Here's how the part is built. I have some questions about the finished solid (model axes, mm). A direction names the side the tool comes from. Coordinates: 2 decimals unless noted, no trailing zeros. Loops run counter-clockwise (first coordinate to the right, second up) from the corner with the lowest first, then second, coordinate; pieces in that order, holes last. Notation, with made-up numbers: (13, 83) - (45, 83) arc R31 cw to (45, 118) - close; hole circle Ø2 at (-13.75, -16.5). An arc over 180 degrees is marked (long way). Use a Markdown table: item, result.
```python
from build123d import *

# Parameters (mm, degrees)
SKETCH_1_W               = 60
SKETCH_1_H               = 3
EXTRUDE_1_DEPTH          = 65
SKETCH_2_W               = 40
SKETCH_2_H               = 3.5
EXTRUDE_2_DEPTH          = 46
EXTRUDE_3_DEPTH          = 3.5
SKETCH_5_W               = 35
SKETCH_5_H               = 17
EXTRUDE_4_DEPTH          = 3
EXTRUDE_START            = 3
SKETCH_6_W               = 35
SKETCH_6_H               = 17
SKETCH_6_W_2             = 20
SKETCH_6_H_2             = 3.5
EXTRUDE_5_DEPTH          = 3
SKETCH_7_W               = 36
SKETCH_7_H               = 10
SKETCH_7_W_2             = 10
SKETCH_7_H_2             = 65
EXTRUDE_6_DEPTH          = 60
SKETCH_8_W               = 66
SKETCH_8_H               = 111
EXTRUDE_7_DEPTH          = 10
SKETCH_9_W               = 15
SKETCH_9_H               = 10
EXTRUDE_8_DEPTH          = 110
SKETCH_10_W              = 36
SKETCH_10_H              = 70
CUT_EXTRUDE_2_DEPTH      = 15
SKETCH_13_W              = 221
SKETCH_13_H              = 10
EXTRUDE_9_DEPTH          = 10
SKETCH_14_W              = 221
SKETCH_14_H              = 10
EXTRUDE_10_DEPTH         = 10
SKETCH_15_W              = 86
SKETCH_15_H              = 10
EXTRUDE_11_DEPTH         = 10
CHAMFER_1_SIZE           = 30
CHAMFER_2_SIZE           = 30
CUT_EXTRUDE_3_DEPTH      = 15
CUT_EXTRUDE_3_DEPTH_BACK = 75
SKETCH_16_R              = 2.1
CHAMFER_3_SIZE           = 5


with BuildPart() as part:
    # 草图1 → 凸台-拉伸1 (new body)
    with BuildSketch(Plane.XY):
        with Locations((0, -32)):
            Rectangle(SKETCH_1_W, SKETCH_1_H)
        with BuildLine():
            Line((-20, -24), (-20, -28))
            Line((-20, -28), (-20, -30))
            Line((-20, -30), (20, -30))
            Line((20, -30), (20, -28))
            Line((20, -28), (20, -24))
            ThreePointArc((20, -24), (21.171572875, -21.171572875), (24, -20))
            Line((24, -20), (28, -20))
            Line((28, -20), (30, -20))
            Line((30, -20), (30, -30.5))
            Line((30, -30.5), (-30, -30.5))
            Line((-30, -30.5), (-30, -20))
            Line((-30, -20), (-28, -20))
            Line((-28, -20), (-24, -20))
            ThreePointArc((-24, -20), (-21.171572875, -21.171572875), (-20, -24))
        make_face()
    extrude(amount=EXTRUDE_1_DEPTH)

    # 草图2 → 凸台-拉伸2 (add)
    with BuildSketch(Plane(origin=(0, 0, 0), x_dir=(-1, 0, 0), z_dir=(0, 0, -1))):
        with Locations((0, -31.75)):
            Rectangle(SKETCH_2_W, SKETCH_2_H)
    extrude(amount=EXTRUDE_2_DEPTH)

    # 草图4 → 凸台-拉伸3 (add)
    with BuildSketch(Plane.XZ.offset(33.5)):
        Polygon((20, -46), (30, -46), (30, -26), (20, -26), (-30, -26), (-30, -46), align=None)
    extrude(amount=-EXTRUDE_3_DEPTH)

    # 草图5 → 凸台-拉伸4 (add)
    with BuildSketch(Plane.ZY.offset(30)):
        with BuildLine():
            Line((-46, -26.5), (-46, -33.5))
            Line((-46, -33.5), (-26, -33.5))
            Line((-26, -33.5), (-26, 8.5))
            Line((-26, 8.5), (56.193548387, -33.5))
            Line((56.193548387, -33.5), (65, -20))
            Line((65, -20), (-26, 26.5))
            Line((-26, 26.5), (-96, 26.5))
            ThreePointArc((-96, 26.5), (-105, 17.5), (-96, 8.5))
            Line((-96, 8.5), (-96, -8.5))
            ThreePointArc((-96, -8.5), (-105, -17.5), (-96, -26.5))
            Line((-96, -26.5), (-46, -26.5))
        make_face()
        with Locations((-63.5, 0)):
            Rectangle(SKETCH_5_W, SKETCH_5_H, mode=Mode.SUBTRACT)
    extrude(amount=EXTRUDE_4_DEPTH)

    # 草图6 → 凸台-拉伸5 (add)
    # profile 1 of 3: a face of its own
    with BuildSketch(Plane(origin=(30, 0, 0), x_dir=(0, 0, -1), z_dir=(1, 0, 0)).offset(EXTRUDE_START)):
        Polygon((26, 8.5), (26, 26.5), (-65, -20), (-56.193548387, -33.5), align=None)
    # profile 2 of 3: a face of its own
    with BuildSketch(Plane(origin=(30, 0, 0), x_dir=(0, 0, -1), z_dir=(1, 0, 0)).offset(EXTRUDE_START)):
        with BuildLine():
            Line((96, 26.5), (46, 26.5))
            Line((46, 26.5), (26, 26.5))
            Line((26, 26.5), (26, 8.5))
            Line((26, 8.5), (26, -30))
            Line((26, -30), (46, -30))
            Line((46, -30), (46, -26.5))
            Line((46, -26.5), (96, -26.5))
            ThreePointArc((96, -26.5), (105, -17.5), (96, -8.5))
            Line((96, -8.5), (96, 8.5))
            ThreePointArc((96, 8.5), (105, 17.5), (96, 26.5))
        make_face()
        with Locations((63.5, 0)):
            Rectangle(SKETCH_6_W, SKETCH_6_H, mode=Mode.SUBTRACT)
    # profile 3 of 3: a face of its own
    with BuildSketch(Plane(origin=(30, 0, 0), x_dir=(0, 0, -1), z_dir=(1, 0, 0)).offset(EXTRUDE_START)):
        with Locations((36, -31.75)):
            Rectangle(SKETCH_6_W_2, SKETCH_6_H_2)
    extrude(amount=-EXTRUDE_5_DEPTH)

    # 草图7 → 凸台-拉伸6 (add)
    with BuildSketch(Plane.XZ.offset(33.5)):
        with Locations((0, -41)):
            Rectangle(SKETCH_7_W, SKETCH_7_H)
        with Locations((-25, 32.5)):
            Rectangle(SKETCH_7_W_2, SKETCH_7_H_2)
        with Locations((25, 32.5)):
            Rectangle(SKETCH_7_W_2, SKETCH_7_H_2)
    extrude(amount=EXTRUDE_6_DEPTH)

    # 草图8 → 凸台-拉伸7 (add)
    with BuildSketch(Plane.XZ.offset(93.5)):
        with Locations((0, 9.5)):
            Rectangle(SKETCH_8_W, SKETCH_8_H)
    extrude(amount=EXTRUDE_7_DEPTH)

    # 草图9 → 凸台-拉伸8 (add)
    with BuildSketch(Plane(origin=(0, 0, -46), x_dir=(-1, 0, 0), z_dir=(0, 0, -1))):
        with Locations((25.5, -98.5)):
            Rectangle(SKETCH_9_W, SKETCH_9_H)
        with Locations((-25.5, -98.5)):
            Rectangle(SKETCH_9_W, SKETCH_9_H)
    extrude(amount=EXTRUDE_8_DEPTH)

    # 草图10 → 切除-拉伸2 (cut)
    with BuildSketch(Plane(origin=(0, 0, -46), x_dir=(-1, 0, 0), z_dir=(0, 0, -1))):
        with Locations((0, -68.5)):
            Rectangle(SKETCH_10_W, SKETCH_10_H)
    extrude(amount=-CUT_EXTRUDE_2_DEPTH, mode=Mode.SUBTRACT)

    # 草图13 → 凸台-拉伸9 (add)
    with BuildSketch(Plane.ZY.offset(33)):
        with Locations((-45.5, -98.5)):
            Rectangle(SKETCH_13_W, SKETCH_13_H)
    extrude(amount=EXTRUDE_9_DEPTH)

    # 草图14 → 凸台-拉伸10 (add)
    with BuildSketch(Plane(origin=(33, 0, 0), x_dir=(0, 0, -1), z_dir=(1, 0, 0))):
        with Locations((45.5, -98.5)):
            Rectangle(SKETCH_14_W, SKETCH_14_H)
    extrude(amount=EXTRUDE_10_DEPTH)

    # 草图15 → 凸台-拉伸11 (add)
    with BuildSketch(Plane.XY.offset(65)):
        with Locations((0, -98.5)):
            Rectangle(SKETCH_15_W, SKETCH_15_H)
    extrude(amount=EXTRUDE_11_DEPTH)

    # 倒角1
    chamfer_1_edges = [part.edges().sort_by_distance(p)[0] for p in [
        (25, -93.5, 0),
    ]]
    chamfer(chamfer_1_edges, length=CHAMFER_1_SIZE)

    # 倒角2
    chamfer_2_edges = [part.edges().sort_by_distance(p)[0] for p in [
        (-25, -93.5, 0),
    ]]
    chamfer(chamfer_2_edges, length=CHAMFER_2_SIZE)

    # 草图16 → 切除-拉伸3 (cut, two sides: drawn at the far end of the back side and taken through both)
    with BuildSketch(Plane(origin=(33, 0, 0), x_dir=(0, 0, -1), z_dir=(1, 0, 0)).offset(-CUT_EXTRUDE_3_DEPTH_BACK)):
        with Locations((93.5, 17.5)):
            Circle(SKETCH_16_R)
        with Locations((58.5, 17.5)):
            Circle(SKETCH_16_R)
        with Locations((58.5, -17.5)):
            Circle(SKETCH_16_R)
        with Locations((93.5, -17.5)):
            Circle(SKETCH_16_R)
    extrude(amount=CUT_EXTRUDE_3_DEPTH + CUT_EXTRUDE_3_DEPTH_BACK, mode=Mode.SUBTRACT)

    # 倒角3
    chamfer_3_edges = [part.edges().sort_by_distance(p)[0] for p in [
        (-18, -98.5, -156),
        (18, -98.5, -156),
        (-43, -98.5, -156),
        (43, -98.5, -156),
        (-43, -98.5, 75),
        (43, -98.5, 75),
    ]]
    chamfer(chamfer_3_edges, length=CHAMFER_3_SIZE)


solid = part.part
```
Q1. If we mould it in two halves opening along Y, with no side actions, what happens to faces 4 (the face through (-31.52, 19.27, -59.63)), 5 (the face through (31.521, 3.575, 18.863)), 6 (the face through (31.521, -26.656, 60.658)), 7 (the face through (20, -27, 32))? For each: pulls with the +Y half, pulls with the -Y half, needs draft (parallel to the pull), parting line crosses it, or undercut.
Check values:
| item | result |
|---|---|
| face 4 | undercut |
| face 5 | pulls with the +Y half |
| face 6 | undercut |
| face 7 | needs draft |
Q2. Which directions (+Z, -Z, +X, -X, +Y, -Y) give clear straight access to the entire face, cutting with the end or side of a thin tool? Please do faces 1 (the face through (-20, -27, 32)), 2 (the face through (30, -57, 27)), 3 (the face through (-30, -1, -40)).
Check values:
| item | result |
|---|---|
| face 1 | +Z, -Z, +Y |
| face 2 | +X |
| face 3 | -Z, +Y |
Q3. I want a section at A-A, the plane x = -9. Write out the boundary of the cut face in (y, z), then the cut area to 3 significant figures.
Check values:
| item | result |
|---|---|
| outline | (-103.5, -31) - (-93.5, -31) - (-93.5, 75) - (-103.5, 75) - close; (-33.5, -46) - (-30, -46) - (-30, 65) - (-33.5, 65) - close |
| area | 1,450 mm^2 |
Q4. Will these pins go through, and if not, where does the flat tip stop? P1, Ø1, axis at x = 23.5, z = 6.5, coming from the +Y side; P2, Ø22, axis at y = -64, z = -5, coming from the -X side; P3, Ø3, axis at x = 27.5, z = -92.5, coming from the +Y side.
Check values:
| item | result |
|---|---|
| P1 | y = -20 |
| P2 | x = -30 |
| P3 | y = -93.5 |
Q5. I want a section at B-B, the plane y = 1. Write out the boundary of the cut face in (x, z).
Check values:
| item | result |
|---|---|
| outline | (-33, -96) - (-30, -96) - (-30, -81) - (-33, -81) - close; (-33, -46) - (-30, -46) - (-30, -26) - (-33, -26) - close; (-33, -11.32) - (-30, -11.32) - (-30, 23.9) - (-33, 23.9) - close; (30, -96) - (33, -96) - (33, -81) - (30, -81) - close; (30, -46) - (33, -46) - (33, -26) - (30, -26) - close; (30, -11.32) - (33, -11.32) - (33, 23.9) - (30, 23.9) - close |
Q6. I want a section at C-C, the plane z = -134.5. Write out the boundary of the cut face in (x, y).
Check values:
| item | result |
|---|---|
| outline | (-43, -103.5) - (-18, -103.5) - (-18, -93.5) - (-43, -93.5) - close; (18, -103.5) - (43, -103.5) - (43, -93.5) - (18, -93.5) - close |
Q7. Please list where these lines run through material, in increasing order: L1, parallel to Y at x = 31.45, z = -58.5; L2, parallel to Y at x = -32.25, z = -93.5; L3, parallel to Y at x = 18, z = -18. Write a range as from..to.
Check values:
| item | result |
|---|---|
| L1 | -103.5..-93.5, -26.5..-19.6, -15.4..-8.5, 8.5..15.4, 19.6..26.5 |
| L2 | -103.5..-93.5, -26.5..-19.6, -15.4..15.4, 19.6..26.5 |
| L3 | -103.5..-93.5, -33.5..-30 |
